from build123d import *

# Parameters (mm, degrees)
EXTRUDE_1_DEPTH     = 100
SKETCH_2_R          = 2.5
CUT_EXTRUDE_1_DEPTH = 124.693168769
SKETCH_3_W          = 20
SKETCH_3_H          = 80
SKETCH_3_W_2        = 50
CUT_EXTRUDE_2_DEPTH = 35
SKETCH_4_W          = 70
SKETCH_4_H          = 100
CUT_EXTRUDE_3_DEPTH = 35
SKETCH_5_W          = 13.228756555
SKETCH_5_H          = 5
CUT_EXTRUDE_4_DEPTH = 124.693168769
SKETCH_7_R          = 2.5
CUT_EXTRUDE_5_DEPTH = 127.984250992
SKETCH_8_W          = 50
SKETCH_8_H          = 80.000000001
CUT_EXTRUDE_7_DEPTH = 20
SKETCH_10_W         = 20
SKETCH_10_H         = 100
EXTRUDE_6_DEPTH     = 5
SKETCH_11_W         = 70
SKETCH_11_H         = 20
EXTRUDE_7_DEPTH     = 5
SKETCH_12_W         = 70
SKETCH_12_H         = 20
EXTRUDE_8_DEPTH     = 5
SKETCH_13_R         = 55
CUT_EXTRUDE_8_DEPTH = 5
SKETCH_14_W         = 10
SKETCH_14_H         = 20
CUT_EXTRUDE_9_DEPTH = 5


with BuildPart() as part:
    # 草图1 → 凸台-拉伸1 (new body)
    with BuildSketch(Plane.XY):
        with BuildLine():
            Line((-50, 20), (50, 20))
            ThreePointArc((50, 20), (70, 0), (50, -20))
            Line((50, -20), (-50, -20))
            ThreePointArc((-50, -20), (-70, 0), (-50, 20))
        make_face()
    extrude(amount=EXTRUDE_1_DEPTH)

    # 草图2 → 切除-拉伸1 (cut, through all)
    with BuildSketch(Plane.XY.offset(100)):
        with Locations((-50, 0)):
            Circle(SKETCH_2_R)
    extrude(amount=-CUT_EXTRUDE_1_DEPTH, mode=Mode.SUBTRACT)

    # 草图3 → 切除-拉伸2 (cut)
    with BuildSketch(Plane.XZ.offset(20)):
        with Locations((-60, 50)):
            Rectangle(SKETCH_3_W, SKETCH_3_H)
        with Locations((-25, 50)):
            Rectangle(SKETCH_3_W_2, SKETCH_3_H)
    extrude(amount=-CUT_EXTRUDE_2_DEPTH, mode=Mode.SUBTRACT)

    # 草图4 → 切除-拉伸3 (cut)
    with BuildSketch(Plane(origin=(0, 20, 0), x_dir=(1, 0, 0), z_dir=(0, 1, 0))):
        with Locations((35, -50)):
            Rectangle(SKETCH_4_W, SKETCH_4_H)
    extrude(amount=-CUT_EXTRUDE_3_DEPTH, mode=Mode.SUBTRACT)

    # 草图5 → 切除-拉伸4 (cut, through all)
    with BuildSketch(Plane.XY.offset(100)):
        with Locations((56.614378278, -17.5)):
            Rectangle(SKETCH_5_W, SKETCH_5_H)
    extrude(amount=-CUT_EXTRUDE_4_DEPTH, mode=Mode.SUBTRACT)

    # 草图7 → 切除-拉伸5 (cut, through all)
    with BuildSketch(Plane(origin=(0, -15, 0), x_dir=(1, 0, 0), z_dir=(0, 1, 0))):
        with Locations(Location((35, -50, 0), (0, 0, 180))):
            Circle(SKETCH_7_R)
    extrude(amount=-CUT_EXTRUDE_5_DEPTH, mode=Mode.SUBTRACT)

    # 草图8 → 切除-拉伸7 (cut)
    with BuildSketch(Plane(origin=(0, 20, 0), x_dir=(1, 0, 0), z_dir=(0, 1, 0))):
        with Locations((-25, -50.000000001)):
            Rectangle(SKETCH_8_W, SKETCH_8_H)
    extrude(amount=-CUT_EXTRUDE_7_DEPTH, mode=Mode.SUBTRACT)

    # 草图10 → 凸台-拉伸6 (add)
    with BuildSketch(Plane(origin=(0, -15, 0), x_dir=(1, 0, 0), z_dir=(0, 1, 0))):
        with Locations((60, -50)):
            Rectangle(SKETCH_10_W, SKETCH_10_H)
    extrude(amount=-EXTRUDE_6_DEPTH)

    # 草图11 → 凸台-拉伸7 (add)
    with BuildSketch(Plane(origin=(0, -20, 0), x_dir=(-1, 0, 0), z_dir=(0, -1, 0))):
        with Locations((-35, 10)):
            Rectangle(SKETCH_11_W, SKETCH_11_H)
    extrude(amount=-EXTRUDE_7_DEPTH)

    # 草图12 → 凸台-拉伸8 (add)
    with BuildSketch(Plane.XZ.offset(20)):
        with Locations((35, 110)):
            Rectangle(SKETCH_12_W, SKETCH_12_H)
    extrude(amount=-EXTRUDE_8_DEPTH)

    # 草图13 → 切除-拉伸8 (cut)
    with BuildSketch(Plane.XZ.offset(20)):
        with Locations((70, 50)):
            Circle(SKETCH_13_R)
    extrude(amount=-CUT_EXTRUDE_8_DEPTH, mode=Mode.SUBTRACT)

    # 草图14 → 切除-拉伸9 (cut)
    with BuildSketch(Plane.XZ.offset(20)):
        with Locations((5, -10)):
            Rectangle(SKETCH_14_W, SKETCH_14_H)
    extrude(amount=-CUT_EXTRUDE_9_DEPTH, mode=Mode.SUBTRACT)


solid = part.part
The listing builds one solid part. Answer for the finished solid, in the listing's coordinates (mm). A direction names the side the tool comes from. Coordinates: 2 decimals unless noted, no trailing zeros. Order: outer loops, then holes, each group sorted by start corner. A loop starts at its lowest first (then second) coordinate and runs counter-clockwise, first axis right, second up.
Q1. A cutting plane is placed at C-C, the plane x = 26. Write down the section's boundary in (y, z).
Q2. Given P1, Ø5.5, axis at y = -17.5, z = -13, coming from the -X side; P2, Ø1.5, axis at y = 18, z = 51, coming from the +X side; P3, Ø6.5, axis at x = -50, y = 0, coming from the -Z side; P4, Ø6, axis at x = 12.5, y = -10, coming from the -Z side, each flat-ended and moving along its own axis, determine where each tip first touches the part or whether it passes through.
Q3. Consider line 1 (Y direction, x = -50, z = 95.25); line 2 (Z direction, x = -60, y = -15); line 3 (X direction, y = 0, z = 7). Determine where each line is inside the solid, lowest interval first.
Q4. A cutting plane is placed at B-B, the plane y = 0. Write down the section's boundary in (x, z), and give its area (3 significant figures).
Q5. A cutting plane is placed at D-D, the plane y = 9.5. Write down the section's boundary in (x, z), and give its area (3 significant figures).
Q6. A cutting plane is placed at A-A, the plane z = 50. Write down the section's boundary in (x, y).
Q7. For a pull along Z with two mould halves and no side action, classify faces 6 (the face through (-50, 18, 51)), 7 (the face through (0, 3, 95)), 8 (the face through (40, -18, -20)) as pulls with the +Z half, pulls with the -Z half, needs draft (parallel to the pull), parting line crosses it, or undercut.
Q8. Which of the six approach directions +Z, -Z, +X, -X, +Y, -Y give full straight-line access (tool end or side, diameter ignored) to faces 1 (the face through (11, -15, 51)), 2 (the face through (0, -18, 49)), 3 (the face through (-25, 20, 95)), 4 (the face through (0, -18, 110)), 5 (the face through (-57, 15, 51))?
Answers follow:
1. outline: (-20, -20) - (-15, -20) - (-15, 17) - (-20, 17) - close; (-20, 83) - (-15, 83) - (-15, 120) - (-20, 120) - close
2. P1: stops at x = 10
2. P2: stops at x = -50
2. P3: stops at z = 0
2. P4: passes through
3. line 1: y = -20 to -2.5, 2.5 to 20
3. line 2: z = 0 to 10, 90 to 100
3. line 3: x = -70 to -52.5, -47.5 to 0
4. outline: (-70, 0) - (-52.5, 0) - (-52.5, 10) - (-70, 10) - close; (-70, 90) - (-52.5, 90) - (-52.5, 100) - (-70, 100) - close; (-47.5, 0) - (0, 0) - (0, 10) - (-47.5, 10) - close; (-47.5, 90) - (0, 90) - (0, 100) - (-47.5, 100) - close
4. area: 1,300 mm2
5. outline: (-67.6, 0) - (0, 0) - (0, 10) - (-67.6, 10) - close; (-67.6, 90) - (0, 90) - (0, 100) - (-67.6, 100) - close
5. area: 1,350 mm2
6. outline: (-63.23, 15) - (-50, 15) - (-50, 20) arc R20 ccw to start; (0, -20) - (15, -20) - (15, -15) - (0, -15) - close
7. face 6: undercut
7. face 7: needs draft
7. face 8: pulls with the -Z half
8. face 1: +Z, -Z, +X, +Y
8. face 2: -X, +Y, -Y
8. face 3: +Z, -Z, +X, -X, +Y
8. face 4: +Z, -X, +Y, -Y
8. face 5: +X, -X, -Y
